Source: CAD feature listing. Evaluate the final solid. Frame: model axes, mm. A direction names the side the tool comes from. Give positions to 0.01 mm unless a question says otherwise; leave off trailing zeros. Loops run counter-clockwise (first coordinate to the right, second up) from the corner with the lowest first, then second, coordinate; pieces in that order, holes last. Notation, with made-up numbers: M 48.25,46.5 L 78.25,46.5 A26 cw 78.25,80.5 Z; hole C -3.5,-10.75 d8. An arc over 180 degrees is marked long. Write item = value, one per line.
from build123d import *

# Parameters (mm, degrees)
F0_W     = 126
F0_H     = 36
F0_W_2   = 106
F0_H_2   = 16
F1_DEPTH = 3
F2_W     = 112
F2_H     = 22
F2_W_2   = 106
F2_H_2   = 16
F3_DEPTH = 50
F4_R     = 5


with BuildPart() as f1:
    # F0 (on Top) → F1 (new body)
    with BuildSketch(Plane.XY):
        with Locations((-53, 8)):
            Rectangle(F0_W, F0_H)
        with Locations((-53, 8)):
            Rectangle(F0_W_2, F0_H_2, mode=Mode.SUBTRACT)
    extrude(amount=F1_DEPTH)

    # F2 (on face) → F3 (join)
    with BuildSketch(Plane.XY.offset(3)):
        with Locations((-53, 8)):
            Rectangle(F2_W, F2_H)
        with Locations((-53, 8)):
            Rectangle(F2_W_2, F2_H_2, mode=Mode.SUBTRACT)
    extrude(amount=F3_DEPTH)

    # F4
    f4_edges = [f1.edges().sort_by_distance(p)[0] for p in [
        (-116, 26, 1.5),
        (10, 26, 1.5),
        (10, -10, 1.5),
        (-116, -10, 1.5),
        (-106, 16, 26.5),
        (0, 16, 26.5),
        (0, 0, 26.5),
        (-106, 0, 26.5),
    ]]
    fillet(f4_edges, radius=F4_R)


solid = f1.part
1. Cut plane A-A, the plane x = -49.5. Return the cut outline in (y, z), then the cut area to 3 significant figures.
Derived:
outline = M -10,0 L 0,0 L 0,53 L -3,53 L -3,3 L -10,3 Z; M 16,0 L 26,0 L 26,3 L 19,3 L 19,53 L 16,53 Z
area = 360 mm²
2. Material intervals for probe 1 along Y at (x, z) = (-39, 36.5); probe 2 along X at (y, z) = (7.5, 32); probe 3 along X at (y, z) = (0.5, 16.5), sorted ascending. Write a range as from..to.
Derived:
probe_1 = -3..0, 16..19
probe_2 = -109..-106, 0..3
probe_3 = -109..-103.18, -2.82..3
3. Cut plane C-C, the plane z = 43.5. Return the cut outline in (x, y).
Derived:
outline = M -109,-3 L 3,-3 L 3,19 L -109,19 Z; hole M -106,5 A5 ccw -101,0 L -5,0 A5 ccw 0,5 L 0,11 A5 ccw -5,16 L -101,16 A5 ccw -106,11 Z
4. Pull-direction query (Y, two-part tool) for faces 1 (the cylindrical face through (-105, 14, 26)), 2 (the flat face through (3, 8, 28)), 3 (the flat face through (0, 8, 26)), 4 (the flat face through (-54, 26, 1)); classes: +Y half, -Y half, draft (parallel to the pull), parting line (faces both ways), or undercut.
Derived:
face_1 = undercut
face_2 = draft
face_3 = undercut
face_4 = +Y half
5. Cut plane B-B, the plane y = 7. Return the cut outline in (x, z).
Derived:
outline = M -116,0 L -106,0 L -106,53 L -109,53 L -109,3 L -116,3 Z; M 0,0 L 10,0 L 10,3 L 3,3 L 3,53 L 0,53 Z
6. Cut plane D-D, the plane y = 23. Return the cut outline in (x, z), then the cut area to 3 significant figures.
Derived:
outline = M -115.58,0 L 9.58,0 L 9.58,3 L -115.58,3 Z
area = 375 mm²
7. Reachability of faces 5 (the cylindrical face through (-105, 2, 27)), 6 (the flat face through (-53.9, 16.3, 0)), 7 (the flat face through (-54, -3, 28)), 8 (the flat face through (-109, 8, 28)), 9 (the cylindrical face through (9, 24, 2)) from +Z, -Z, +X, -X, +Y, -Y: full face, straight path, thin tool, end or side. Return the list, or none.
Derived:
face_5 = +Z, -Z
face_6 = -Z, +X, -X, +Y, -Y
face_7 = +Z, +X, -X, -Y
face_8 = +Z, -X, +Y, -Y
face_9 = +Z, -Z, +X, +Y
8. First-contact query: pin 1 Ø1 at (y, z) = (8, 26) entering from -X; pin 2 Ø4 at (x, z) = (-77, 27.5) entering from +Y; pin 3 Ø5 at (y, z) = (11, 33) entering from +X; pin 4 Ø1.5 at (x, y) = (-83, 1.5) entering from +Z. Flat tips, straight axial feed; report the tip coordinate or a pass-through.
Derived:
pin_1 = -109
pin_2 = 19
pin_3 = 3
pin_4 = through
